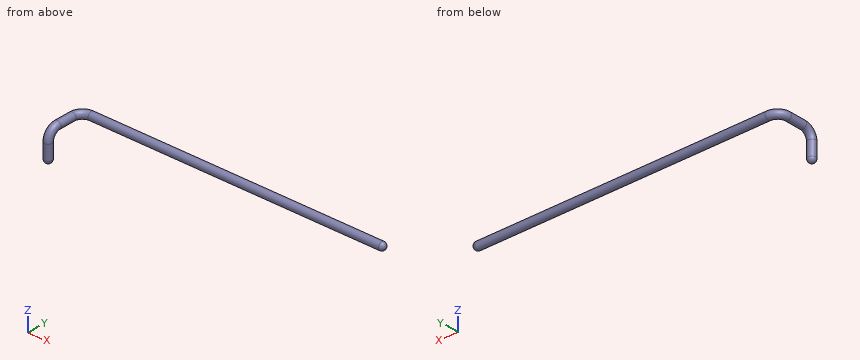
```python
from build123d import *

# Parameters (mm, degrees)
SKICA4_R                       = 0.575
T_HNOUT_PO_K_IVCE2_OUTLINE_R   = 0.575
T_HNOUT_PO_K_IVCE2_ANGLE       = 90
T_HNOUT_START                  = -0.2500001
T_HNOUT_PO_K_IVCE2_2_OUTLINE_R = 0.575
T_HNOUT_PO_K_IVCE2_2_DEPTH     = 2.5000002
T_HNOUT_START_2                = -4.25
T_HNOUT_PO_K_IVCE2_3_OUTLINE_R = 0.575
T_HNOUT_PO_K_IVCE2_3_DEPTH     = 2.7500001
ZAOBLIT1_R                     = 0.575


with BuildPart() as part:
    # Táhnout po křivce1: sweep along a path in Skica1
    with BuildLine(Plane.XY) as t_hnout_po_k_ivce1_path:
        Line((0, 0), (0, 2.25))
        ThreePointArc((0, 2.25), (0.439339828, 3.310660172), (1.5, 3.75))
        Line((1.5, 3.75), (45, 3.75))
    # Skica4 → Táhnout po křivce1 (sweep)
    with BuildSketch(Plane(origin=(45, 0, 0), x_dir=(0, 0, -1), z_dir=(1, 0, 0))):
        with Locations((0, 3.75)):
            Circle(SKICA4_R)
    sweep(path=t_hnout_po_k_ivce1_path.line)



with BuildPart() as body_2:
    # Táhnout po křivce2: read off the stored shape, not the designer's step
    # Táhnout po křivce2 outline → Táhnout po křivce2 (revolve)
    with BuildSketch(Plane(origin=(0, -0.25, -1.5), x_dir=(0, 0, 1), z_dir=(0, 1, 0))):
        with Locations((1.5, 0)):
            Circle(T_HNOUT_PO_K_IVCE2_OUTLINE_R)
    revolve(axis=Axis((0, -0.25, -1.5), (1, 0, 0)), revolution_arc=T_HNOUT_PO_K_IVCE2_ANGLE)


with BuildPart() as part_1:
    add(part.part)

    add(body_2.part)  # T_hnout po k_ivce2 2 merges body 2
    # T_hnout po k_ivce2 2 outline → T_hnout po k_ivce2 2 (add)
    with BuildSketch(Plane(origin=(0, 0, 0), x_dir=(1, 0, 0), z_dir=(0, 1, 0)).offset(T_HNOUT_START)):
        Circle(T_HNOUT_PO_K_IVCE2_2_OUTLINE_R)
    extrude(amount=T_HNOUT_PO_K_IVCE2_2_DEPTH)

    # T_hnout po k_ivce2 3 outline → T_hnout po k_ivce2 3 (add)
    with BuildSketch(Plane.XY.offset(T_HNOUT_START_2)):
        with Locations((0, -1.75)):
            Circle(T_HNOUT_PO_K_IVCE2_3_OUTLINE_R)
    extrude(amount=T_HNOUT_PO_K_IVCE2_3_DEPTH)

    # Zaoblit1
    zaoblit1_edges = [part_1.edges().sort_by_distance(p)[0] for p in [
        (45, 3.75, 0.575),
        (-0.575, -1.75, -4.25),
    ]]
    fillet(zaoblit1_edges, radius=ZAOBLIT1_R)


solid = part_1.part
```
The listing builds one solid part. Answer for the finished solid, in the listing's coordinates (mm). Coordinates: 2 decimals unless noted, no trailing zeros. Loops run counter-clockwise (first coordinate to the right, second up) from the corner with the lowest first, then second, coordinate; pieces in that order, holes last. Notation, with made-up numbers: M 30,50 L 80,50 A21 ccw 80,56 Z; hole C 38,-39.75 d3. An arc over 180 degrees is marked long. Answer as CSV lines item,"result". Start each with the question number.
(1) The part is cut by section B-B (z = -1.95). Give the vertices of the cut face in (x, y) (3 decimals).
(2) Find the intervals of material crossed by L1, parallel to X at y = -1.75, z = -3.3 (3 decimals); L2, parallel to X at y = 2.5, z = 0.3, in increasing order. Write a range as [from, to].
(3) The part is cut by section A-A (x = 40.5). Give the vertices of the cut face in (y, z) (3 decimals), and give its area (3 significant figures).
Determined:
1,outline,"C 0,-1.75 d1.15"
2,L1,"[-0.575, 0.575]"
2,L2,"[-0.47, 0.52]"
3,outline,"C 3.75,0 d1.15"
3,area,"1.04 mm2"
